Geometry: final body of the model. Coordinates: model frame, mm. Face numbers are marked on the shaded views. A direction names the side the tool comes from. Give positions to 0.01 mm unless a question says otherwise; leave off trailing zeros. Loops run counter-clockwise (first coordinate to the right, second up) from the corner with the lowest first, then second, coordinate; pieces in that order, holes last. Notation, with made-up numbers: (-17.75, -20.75) - (32.25, -20.75) arc R18 cw to (32.25, -0.75) - close; hole circle Ø6 at (-25.5, 17.5). An arc over 180 degrees is marked (long way). Answer in a Markdown table with one row per item.
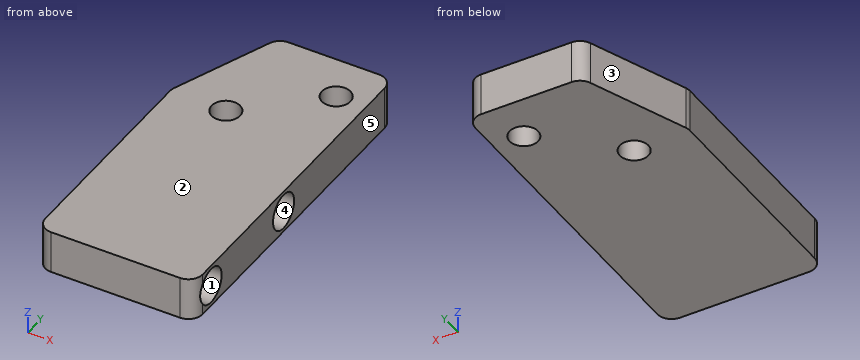
from build123d import *

# Parameters (mm, degrees)
BOSS_EXTRUDE1_DEPTH = 19.05
SKETCH2_R           = 7.9375
CUT_EXTRUDE1_DEPTH  = 15.24
SKETCH3_R           = 6.35
CUT_EXTRUDE3_DEPTH  = 167.433003338
FILLET1_R           = 6.35


with BuildPart() as part:
    # Sketch1 → Boss-Extrude1 (new body)
    with BuildSketch(Plane.XY):
        Polygon((0, 0), (0, -149.86), (-69.85, -149.86), (-69.85, -48.26), (-50.8, 0), align=None)
    extrude(amount=BOSS_EXTRUDE1_DEPTH)

    # Sketch2 → Cut-Extrude1 (cut)
    with BuildSketch(Plane(origin=(0, 0, 0), x_dir=(0, 0, -1), z_dir=(1, 0, 0))):
        with Locations((-9.525, -82.55)):
            Circle(SKETCH2_R)
        with Locations((-9.525, -137.16)):
            Circle(SKETCH2_R)
    extrude(amount=-CUT_EXTRUDE1_DEPTH, mode=Mode.SUBTRACT)

    # Sketch3 → Cut-Extrude3 (cut, through all)
    with BuildSketch(Plane.XY.offset(19.05)):
        with Locations((-45.0596, -49.53)):
            Circle(SKETCH3_R)
        with Locations((-13.3096, -20.32)):
            Circle(SKETCH3_R)
    extrude(amount=-CUT_EXTRUDE3_DEPTH, mode=Mode.SUBTRACT)

    # Fillet1
    # the kernel refuses this fillet: 6.35 mm, written as the material it takes off along each edge
    with BuildSketch(Plane(origin=(0, 0, -15.875), x_dir=(0, -1, 0), z_dir=(0, 0, 1))) as fillet1_piece_1:
        with BuildLine():
            CenterArc((FILLET1_R, -FILLET1_R), FILLET1_R, 90, 90)
            Line((0, -FILLET1_R), (0, 0))
            Line((0, 0), (FILLET1_R, 0))
        make_face()
    extrude(amount=50.8, mode=Mode.SUBTRACT)
    with BuildSketch(Plane(origin=(0, -149.86, -15.875), x_dir=(0, 1, 0), z_dir=(0, 0, 1)), Plane(origin=(-69.85, -149.86, -15.875), x_dir=(1, 0, 0), z_dir=(0, 0, 1))) as fillet1_piece_2:
        with BuildLine():
            CenterArc((FILLET1_R, FILLET1_R), FILLET1_R, 180, 90)
            Line((0, FILLET1_R), (0, 0))
            Line((0, 0), (FILLET1_R, 0))
        make_face()
    extrude(amount=50.8, mode=Mode.SUBTRACT)
    with BuildSketch(Plane(origin=(-69.85, -48.26, -3.019844557), x_dir=(0.367166534736053, 0.9301552213313209, 0), z_dir=(0, 0, 1))) as fillet1_piece_3:
        with BuildLine():
            CenterArc((FILLET1_R * 0.190226428775, -FILLET1_R), FILLET1_R, 90, 21.540975919)
            Line((-FILLET1_R * 0.176940105961, -FILLET1_R * 0.0698447786687), (0, 0))
            Line((0, 0), (FILLET1_R * 0.190226428775, 0))
        make_face()
    extrude(amount=25.089689114, mode=Mode.SUBTRACT)
    with BuildSketch(Plane(origin=(-50.8, 0, -10.800596536), x_dir=(1, 0, 0), z_dir=(0, 0, 1))) as fillet1_piece_4:
        with BuildLine():
            CenterArc((FILLET1_R * 0.680352537675, -FILLET1_R), FILLET1_R, 90, 68.459024081)
            Line((-FILLET1_R * 0.249802683657, -FILLET1_R * 0.632833465264), (0, 0))
            Line((0, 0), (FILLET1_R * 0.680352537675, 0))
        make_face()
    extrude(amount=40.651193071, mode=Mode.SUBTRACT)


solid = part.part
Q1. Cut plane D-D (y = -137.16). Output: boundary loops of the cut face in (x, z).
Check values:
| item | result |
|---|---|
| outline | (-69.85, 0) - (0, 0) - (0, 1.59) - (-15.24, 1.59) - (-15.24, 17.46) - (0, 17.46) - (0, 19.05) - (-69.85, 19.05) - close |
Q2. First-contact query: pin 1 (9.5 mm diameter, centred on y = -137.16, z = 9.525, fed in from +X); pin 2 (2 mm diameter, centred on y = -25.5, z = 7, fed in from +X); pin 3 (6 mm diameter, centred on y = -37, z = 7, fed in from -X); pin 4 (1 mm diameter, centred on y = -24.5, z = 16.5, fed in from -X). Flat tips, straight axial feed; report the tip coordinate or a pass-through.
Check values:
| item | result |
|---|---|
| pin 1 | x = -15.24 |
| pin 2 | x = 0 |
| pin 3 | x = -66.59 |
| pin 4 | x = -60.67 |
Q3. Reachability of the marked faces 4 and 5 from +Z, -Z, +X, -X, +Y, -Y: full face, straight path, thin tool, end or side. Return the list, or none.
Check values:
| item | result |
|---|---|
| face 4 | +X |
| face 5 | +Z, -Z, +X, +Y, -Y |
Q4. Draft query along Z for the marked faces 1, 2 and 3. Return one class per face: pulls with the +Z half, pulls with the -Z half, needs draft (parallel to the pull), parting line crosses it, or undercut.
Check values:
| item | result |
|---|---|
| face 1 | undercut |
| face 2 | pulls with the +Z half |
| face 3 | needs draft |
Q5. Cut plane B-B (x = -49). Output: boundary loops of the cut face in (y, z), and give its area (3 significant figures).
Check values:
| item | result |
|---|---|
| outline | (-149.86, 0) - (-54.51, 0) - (-54.51, 19.05) - (-149.86, 19.05) - close; (-44.55, 0) - (-0.52, 0) - (-0.52, 19.05) - (-44.55, 19.05) - close |
| area | 2,660 mm² |
Q6. Cut plane C-C (z = 11). Output: boundary loops of the cut face in (x, y), and give its area (3 significant figures).
Check values:
| item | result |
|---|---|
| outline | (-69.85, -143.51) arc R6.35 ccw to (-63.5, -149.86) - (-6.35, -149.86) arc R6.35 ccw to (-0.17, -144.96) - (-15.24, -144.96) - (-15.24, -129.36) - (0, -129.36) - (0, -90.35) - (-15.24, -90.35) - (-15.24, -74.75) - (0, -74.75) - (0, -6.35) arc R6.35 ccw to (-6.35, 0) - (-46.48, 0) arc R6.35 ccw to (-52.39, -4.02) - (-69.41, -47.14) arc R6.35 ccw to (-69.85, -49.47) - close; hole circle Ø12.7 at (-45.06, -49.53); hole circle Ø12.7 at (-13.31, -20.32) |
| area | 9,250 mm² |
Q7. Cut plane A-A (y = -20.32). Output: boundary loops of the cut face in (x, z).
Check values:
| item | result |
|---|---|
| outline | (-58.82, 0) - (-19.66, 0) - (-19.66, 19.05) - (-58.82, 19.05) - close; (-6.96, 0) - (0, 0) - (0, 19.05) - (-6.96, 19.05) - close |
Q8. Material intervals for line 1 along Y through (x, z) = (-6, 16.5); line 2 along Y through (x, z) = (-4, 15.5); line 3 along Z through (x, y) = (-11, -137), sorted ascending.
Check values:
| item | result |
|---|---|
| line 1 | -149.85 to -140.95, -133.37 to -86.34, -78.76 to -0.01 |
| line 2 | -149.41 to -142.39, -131.93 to -87.78, -77.32 to -0.45 |
| line 3 | 0 to 1.59, 17.46 to 19.05 |
